Design review of the part built by this model. Coordinates are the model's own, in mm. A direction names the side the tool comes from. Coordinates: 2 decimals unless noted, no trailing zeros. Write each loop counter-clockwise with the first axis right and the second up, starting at its lowest first coordinate (ties: lowest second). Pieces come first, ordered by that corner, then holes.
```python
from build123d import *

# Parameters (mm, degrees)
COPYSKETCH003_W  = 40
COPYSKETCH003_H  = 60
PAD_DEPTH        = 3.5
POCKET_DEPTH     = 1.5
FILLET_R         = 1.5
FILLET001_R      = 1.5
HOLE_D           = 3.3
HOLE_DEPTH       = 25
HOLE_CSINK_D     = 6
HOLE_CSINK_ANGLE = 90


with BuildPart() as part:
    # CopySketch003 → Pad (new body)
    with BuildSketch(Plane.XY):
        Rectangle(COPYSKETCH003_W, COPYSKETCH003_H)
    extrude(amount=PAD_DEPTH)

    # CopySketch002 → Pocket (cut)
    with BuildSketch(Plane.XY.offset(3.5)):
        Polygon((-12.6, 29), (12.6, 29), (12.6, 22.6), (19, 22.6), (19, -22.6), (12.6, -22.6), (12.6, -29), (-12.6, -29), (-12.6, -22.6), (-19, -22.6), (-19, 22.6), (-12.6, 22.6), align=None)
    extrude(amount=-POCKET_DEPTH, mode=Mode.SUBTRACT)

    # Fillet
    fillet_edges = [part.edges().sort_by_distance(p)[0] for p in [
        (20, -30, 1.75),
        (-20, -30, 1.75),
        (20, 30, 1.75),
        (-20, 30, 1.75),
    ]]
    fillet(fillet_edges, radius=FILLET_R)

    # Fillet001
    fillet001_edges = [part.edges().sort_by_distance(p)[0] for p in [
        (0, 30, 0),
        (-19.56066, 29.56066, 0),
        (19.56066, 29.56066, 0),
        (-20, 0, 0),
        (20, 0, 0),
        (-19.56066, -29.56066, 0),
        (19.56066, -29.56066, 0),
        (0, -30, 0),
    ]]
    fillet(fillet001_edges, radius=FILLET001_R)

    # Hole
    with Locations(Plane(origin=(0, 0, 0), x_dir=(1, 0, 0), z_dir=(0, 0, -1))):
        with Locations((15.5, 25.5), (15.5, -25.5), (-15.5, -25.5), (-15.5, 25.5)):
            CounterSinkHole(HOLE_D / 2, HOLE_CSINK_D / 2, depth=HOLE_DEPTH, counter_sink_angle=HOLE_CSINK_ANGLE)


solid = part.part
```
(1) Consider section D-D (x = -14.5). State how many separate pieces and enclosed holes the cut face has, plus the area to 3 significant figures.
(2) Wall thickness on line 1 (X direction, y = 25.5, z = 2.05); line 2 (Y direction, x = 15.5, z = 2.4); line 3 (Y direction, x = 6, z = 2.3): over which ranges is each line inside the solid? List them lowest first.
(3) Consider section B-B (x = -7.5). Give the boundary of the cut face in (y, z).
(4) For faces 1 (the flat face through (0, 30, 2)), 2 (the flat face through (12.6, 26, 3)), list the 3-axis set-ups (+Z, -Z, +X, -X, +Y, -Y) from which the entire face can be reached by the end or side of a thin tool; tool diameter is ignored.
(5) Consider section C-C (y = -17). Give the boundary of the cut face in (x, z), plus the area to 3 significant figures.
(6) Consider section A-A (z = 2.95). Give the boundary of the cut face in (x, y), plus the area to 3 significant figures.
(7) Mouldability with a two-part tool opening along X and no side actions: class faces 3 (the cylindrical face through (-19.57, 29.55, 2.51)), 4 (the cylindrical face through (-0.26, -29.55, 0.43)), 5 (the cylindrical face through (14.61, 24.11, 2.44)) as +X half, -X half, draft (parallel to the pull), parting line (faces both ways), or undercut.
(8) Insertion check: pin 1 Ø11.5 at (x, y) = (-6.5, 9) entering from +Z. The pin has a flat end and moves straight along its axis. Give the tip position at first contact, or say it passes through.
Results:
1. separate pieces: 3
1. enclosed holes: 0
1. area: 119 mm2
2. line 1: x = -20 to -17.15, -13.85 to -12.6, 12.6 to 13.85, 17.15 to 20
2. line 2: y = -30 to -27.15, -23.85 to -22.6, 22.6 to 23.85, 27.15 to 30
2. line 3: y = -30 to -29, 29 to 30
3. outline: (-30, 1.5) arc R1.5 ccw to (-28.5, 0) - (28.5, 0) arc R1.5 ccw to (30, 1.5) - (30, 3.5) - (29, 3.5) - (29, 2) - (-29, 2) - (-29, 3.5) - (-30, 3.5) - close
4. face 1: +Z, -Z, +X, -X, +Y
4. face 2: +Z
5. outline: (-20, 1.5) arc R1.5 ccw to (-18.5, 0) - (18.5, 0) arc R1.5 ccw to (20, 1.5) - (20, 3.5) - (19, 3.5) - (19, 2) - (-19, 2) - (-19, 3.5) - (-20, 3.5) - close
5. area: 82.0 mm2
6. outline: (-20, -28.5) arc R1.5 ccw to (-18.5, -30) - (18.5, -30) arc R1.5 ccw to (20, -28.5) - (20, 28.5) arc R1.5 ccw to (18.5, 30) - (-18.5, 30) arc R1.5 ccw to (-20, 28.5) - close; hole (-19, -22.6) - (-12.6, -22.6) - (-12.6, -29) - (12.6, -29) - (12.6, -22.6) - (19, -22.6) - (19, 22.6) - (12.6, 22.6) - (12.6, 29) - (-12.6, 29) - (-12.6, 22.6) - (-19, 22.6) - close; hole circle Ø3.3 at (-15.5, -25.5); hole circle Ø3.3 at (-15.5, 25.5); hole circle Ø3.3 at (15.5, -25.5); hole circle Ø3.3 at (15.5, 25.5)
6. area: 324 mm2
7. face 3: -X half
7. face 4: draft
7. face 5: undercut
8. pin 1: stops at z = 2
